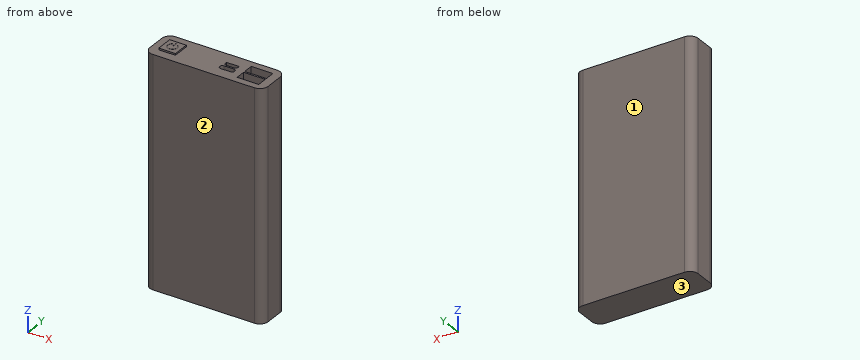
Autodesk Inventor part; units mm, degrees
ref_plane "YZ Plane" through (0, 0, 0) normal (1, 0, 0) x (0, 1, 0)
ref_plane "XZ Plane" through (0, 0, 0) normal (0, 1, 0) x (-1, 0, 0)
ref_plane "XY Plane" through (0, 0, 0) normal (0, 0, 1) x (1, 0, 0)
sketch "Sketch1" plane through (0, 0, 0) normal (0, 1, 0) x (-1, 0, 0)
  line L0 (0, 0) -> (71, 0)
  line L1 (71, 0) -> (71, -137)
  line L2 (71, -137) -> (0, -137)
  line L3 (0, -137) -> (0, 0)
  dimension "d0" = 137
  dimension "d1" = 71
extrude "Extrusion1" add sketch "Sketch1" along normal blind 21
fillet "Fillet1" radius 5 4 edges at (0, 21, -68.5) (0, 0, -68.5) (-71, 21, -68.5) (-71, 0, -68.5)
sketch "Sketch2" plane through (-66, 0, 0) normal (0, 0, 1) x (1, 0, 0)
  line L0 (0, 15.5) -> (10, 15.5)
  line L1 (10, 15.5) -> (10, 5.5)
  line L2 (10, 5.5) -> (0, 5.5)
  line L3 (0, 5.5) -> (0, 15.5)
  line L4 (48, 17) -> (61, 17)
  line L5 (61, 17) -> (61, 11)
  line L6 (61, 11) -> (48, 11)
  line L7 (48, 11) -> (48, 17)
  line L8 (48, 10) -> (61, 10)
  line L9 (61, 10) -> (61, 4)
  line L10 (61, 4) -> (48, 4)
  line L11 (48, 4) -> (48, 10)
  line L12 (66, 5) -> (66, 16)
  line L13 (0, 0) -> (61, 0)
  line L14 (0, 21) -> (61, 21)
  line L15 (-5, 5) -> (-5, 16)
  line L16 (35.4, 13.6) -> (43, 13.6)
  line L17 (43, 13.6) -> (43, 11)
  line L18 (43, 11) -> (35.4, 11)
  line L19 (35.4, 11) -> (35.4, 13.6)
  line L20 (36.2, 10) -> (42.2, 10)
  line L21 (43.7, 8.5) -> (43.7, 8.3)
  line L22 (42.2, 6.8) -> (36.2, 6.8)
  line L23 (34.7, 8.3) -> (34.7, 8.5)
  arc A0 (36.2, 10) -> (34.7, 8.5) centre (36.2, 8.5) ccw
  arc A1 (43.7, 8.5) -> (42.2, 10) centre (42.2, 8.5) ccw
  arc A2 (34.7, 8.3) -> (36.2, 6.8) centre (36.2, 8.3) ccw
  arc A3 (42.2, 6.8) -> (43.7, 8.3) centre (42.2, 8.3) ccw
  line L24 (35.4, 12) -> (36.4, 11)
  line L25 (43, 12) -> (42, 11)
  point P0 (66, 0)
  point P1 (0, 10.5)
  point P2 (-5, 10.5)
  point P3 (43.7, 6.8)
  point P4 (34.7, 6.8)
  point P5 (39.2, 11)
  point P6 (39.2, 10)
  dimension "d5" = 6
  dimension "d6" = 6
  dimension "d7" = 13
  dimension "d8" = 5
  dimension "d9" = 4
  dimension "d10" = 4
  dimension "d11" = 5
  dimension "d12" = 10
  dimension "d13" = 10
  dimension "d14" = 7.6
  dimension "d15" = 2.6
  dimension "d16" = 5
  dimension "d17" = 3.2
  dimension "d19" = 9
  dimension "d20" = 1
  dimension "d21" = 1.5
  dimension "d26" = 45
  dimension "d27" = 45
  dimension "d28" = 1
  dimension "d29" = 1
extrude "Extrusion2" cut sketch "Sketch2" against normal blind 20 contours L4 L5 L6 L7 | L8 L9 L10 L11 | L16 L17 L25 L18 L24 L19 | L20 A1 L21 A3 L22 A2 L23 A0
extrude "Extrusion3" add sketch "Sketch2" along normal blind 1 contours L0 L1 L2 L3
sketch "Sketch3" plane through (-66, 0, 1) normal (0, 0, 1) x (1, 0, 0)
  circle A0 centre (5, 10.5) radius 3 construction
  arc A1 (3.0716, 12.7981) -> (6.9284, 12.7981) centre (5, 10.5) ccw
  line L0 (3.0716, 12.7981) -> (5, 10.5) construction
  line L1 (5, 10.5) -> (6.9284, 12.7981) construction
  line L2 (5, 10.5) -> (5, 13.5) construction
  line L3 (10, 5.5) -> (10, 15.5)
  line L4 (10, 15.5) -> (0, 15.5)
  circle A2 centre (5, 10.5) radius 2.5 construction
  arc A3 (3.393, 12.4151) -> (6.607, 12.4151) centre (5, 10.5) ccw
  arc A4 (3.393, 12.4151) -> (3.0716, 12.7981) centre (3.2323, 12.6066) ccw
  arc A5 (6.9284, 12.7981) -> (6.607, 12.4151) centre (6.7677, 12.6066) ccw
  line L5 (4.75, 14) -> (5.25, 14) construction
  line L6 (5.25, 14) -> (5.25, 11.5)
  line L7 (5.25, 11.5) -> (4.75, 11.5) construction
  line L8 (4.75, 11.5) -> (4.75, 14)
  arc A6 (5.25, 14) -> (4.75, 14) centre (5, 14) ccw
  arc A7 (4.75, 11.5) -> (5.25, 11.5) centre (5, 11.5) ccw
  point P0 (66, 0)
  point P1 (10, 10.5)
  point P2 (5, 15.5)
  dimension "d30" = 40
  dimension "d31" = 40
  dimension "d32" = 6
  dimension "d33" = 0.5
  dimension "d34" = 0.5
  dimension "d35" = 2.5
  dimension "d36" = 1
extrude "Extrusion4" cut sketch "Sketch3" against normal blind 0.1
properties part number "power bank"
Geometry check sheet. Reference: the model listing, model coordinates, mm. Face numbers are marked on the shaded views. Round coordinates to 2 decimals unless told otherwise and drop trailing zeros. Write each question's results on one line, items separated by ' | '.
(1) Sectioned sample at A-A, the plane z = -18. Count the separate pieces of the cut face and the enclosed holes in it, plus the area to 3 significant figures.
Computed:
separate pieces: 1 | enclosed holes: 4 | area: 1,270 mm^2
(2) Thickness scan on probe 1 along X at (y, z) = (8.75, -13); probe 2 along X at (y, z) = (10.5, 0.95); probe 3 along Z at (x, y) = (-6, 12). Record the ranges inside material, lowest first. Write a range as from..to.
Computed:
probe 1: x = -71..-31.28, -22.32..-18, -5..0 | probe 2: x = -66..-64, -63.5..-58.5, -58..-56 | probe 3: z = -137..-20
(3) Depth check by flat-ended pin: pin 1 Ø3 at (x, z) = (-63, -111.5) entering from -Y; pin 2 Ø0.5 at (x, z) = (-60, 0.5) entering from -Y; pin 3 Ø5 at (x, y) = (-30, 16) entering from +Z; pin 4 Ø1.8 at (x, y) = (-12, 7.5) entering from +Z. Enter the tip coordinate at first touch or a pass-through.
Computed:
pin 1: stops at y = 0 | pin 2: stops at y = 5.5 | pin 3: stops at z = 0 | pin 4: stops at z = -20
(4) Draft check along Y on the marked faces 1, 2 and 3. Enter one of: pulls with the +Y half, pulls with the -Y half, needs draft (parallel to the pull), parting line crosses it, or undercut.
Computed:
face 1: pulls with the +Y half | face 2: pulls with the -Y half | face 3: needs draft
